Can you work these out from the model? Positions are in its coordinate system, mm. Round coordinates to 2 decimals unless told otherwise and drop trailing zeros. Order: outer loops, then holes, each group sorted by start corner. A loop starts at its lowest first (then second) coordinate and runs counter-clockwise, first axis right, second up. Notation, with made-up numbers: (6.25, 20) - (44.25, 20) arc R30 cw to (44.25, 47) - close; hole circle Ø5 at (38, -12.5). An arc over 180 degrees is marked (long way). Write item = value, one per line.
from build123d import *

# Parameters (mm, degrees)
F1_DEPTH = 63.5


with BuildPart() as f1:
    # F0 (on Front) → F1 (new body, symmetric)
    with BuildSketch(Plane.XZ):
        Polygon((-25.263004, -11.258429), (-22.252139, -16.426012), (-18.200789, -20.825533), (-13.298391, -24.251275), (-7.774175, -26.543055), (-1.886447, -27.593711), (4.08949, -27.354116), (9.874206, -25.835472), (15.197215, -23.108791), (19.80962, -19.301568), (23.495748, -14.591825), (26.083242, -9.199785), (27.451112, -3.377573), (27.535399, 2.60257), (26.332161, 8.46102), (23.89766, 13.923843), (20.345732, 18.735601), (15.842459, 22.671304), (10.598411, 25.546922), (4.858793, 27.227995), (-1.108017, 27.635916), (-7.023017, 26.751613), (-12.609629, 24.616434), (-17.606628, 21.330218), (-21.780362, 17.046625), (-24.935669, 11.96595), (-26.925013, 6.325761), (-27.655373, 0.389787), (-27.092598, -5.564414), align=None)
    extrude(amount=F1_DEPTH, both=True)


solid = f1.part
(1) Will these pins go through, and if not, where does the flat tip stop? P1, Ø5, axis at x = 15, y = 29, coming from the -Z side; P2, Ø1.5, axis at x = -18, y = -3.5, coming from the +Z side; P3, Ø3, axis at y = 46, z = 6.5, coming from the -X side.
Computed:
P1 = -24.49
P2 = 21.56
P3 = -27.09
(2) If we section it at C-C (x = 8.5): Write out the boundary of the cut face in (y, z).
Computed:
outline = (-63.5, -26.2) - (63.5, -26.2) - (63.5, 26.16) - (-63.5, 26.16) - close
(3) If I drill on line 1 (X direction, y = -38.5, z = 24.5); line 2 (X direction, y = -49.5, z = -23.5); line 3 (Z direction, x = 4.5, y = -22.5), over which ranges is the centre line in solid material (lowest first)? Write a range as from..to.
Computed:
line_1 = -12.79..12.51
line_2 = -14.37..14.43
line_3 = -27.25..27.25
(4) If we section it at B-B (z = 10): Write out the boundary of the cut face in (x, y).
Computed:
outline = (-25.63, -63.5) - (25.65, -63.5) - (25.65, 63.5) - (-25.63, 63.5) - close
